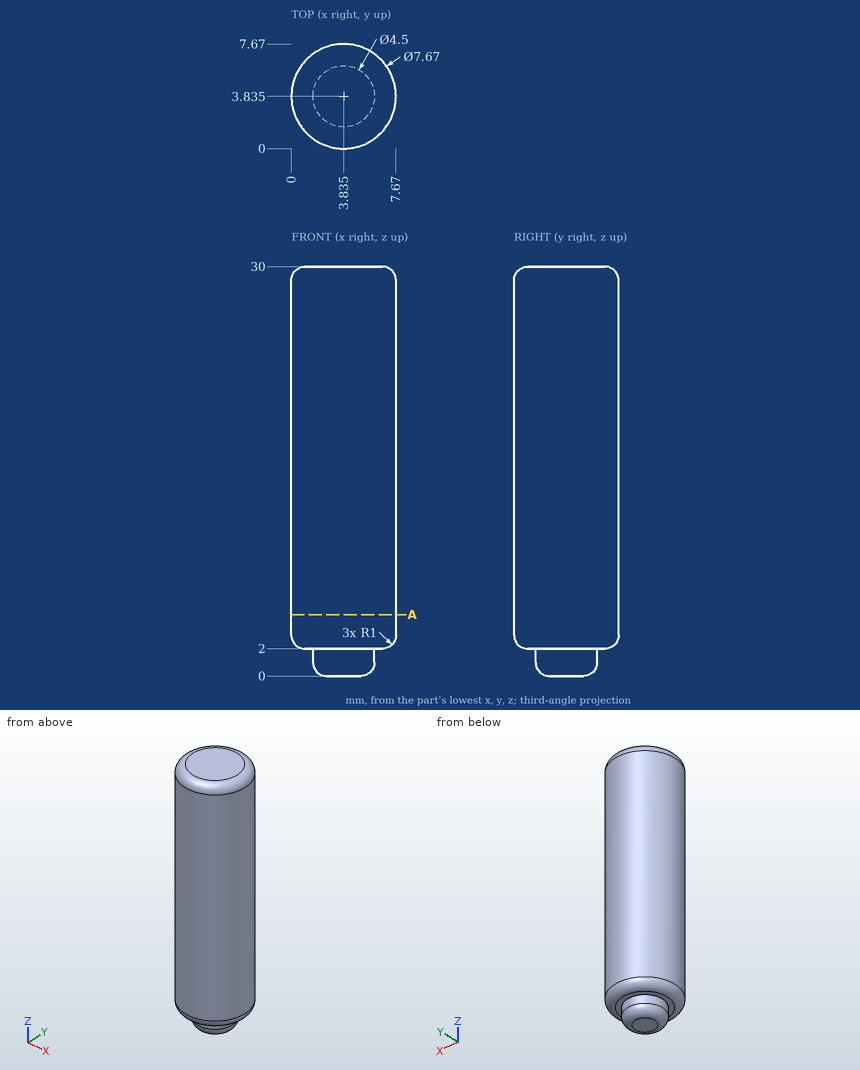
The figure shows three views and two pictorial views of one solid part (mm, origin at its lowest corner). Answer the questions. Coordinates: 2 decimals unless noted, no trailing zeros. Loops run counter-clockwise (first coordinate to the right, second up) from the corner with the lowest first, then second, coordinate; pieces in that order, holes last. Notation, with made-up numbers: (35.25, 16.25) -> (43.25, 16.25) arc R23 ccw to (43.25, 55.25) -> close; hole circle Ø5 at (-24.75, 36.5). An arc over 180 degrees is marked (long way). Use one line per item in the form item = value. Start each with the question number.
Item 1: The part is cut by section A-A on z = 4.5. Determine the outline of the cut face in (x, y) (3 decimals), then the cut area to 3 significant figures.
Item 2: A flat-ended cylindrical pin translates along its axis: pin 1 Ø3 at (y, z) = (4.5, 4.5) entering from +X. Find the tip coordinate at first contact, or state that the pin passes through.
Item 3: Consider L1, parallel to Z at x = 5.25, y = 6; L2, parallel to X at y = 4, z = 1.5; L3, parallel to Y at x = 1.25, z = 22.5. Determine where each line is inside the solid, lowest interval first. Write a range as [from, to].
Answer key:
q1.outline = circle Ø7.67 at (3.835, 3.835)
q1.area = 46.2 mm2
q2.pin_1 = 7.67
q3.L1 = [2, 30]
q3.L2 = [1.59, 6.08]
q3.L3 = [1, 6.67]
